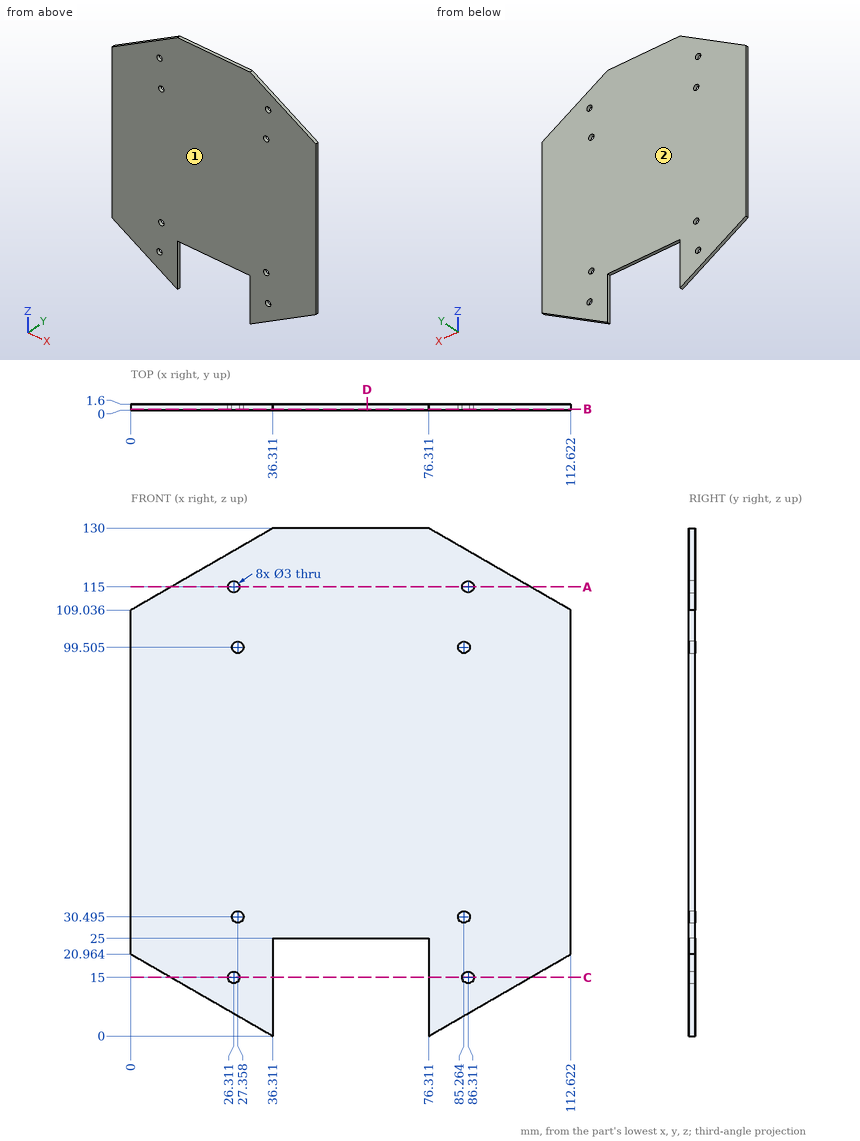
Check sheet for the drawn part. Datum: minimum x, y, z corner. Units: mm. Round coordinates to 2 decimals unless told otherwise and drop trailing zeros. Order: outer loops, then holes, each group sorted by start corner. A loop starts at its lowest first (then second) coordinate and runs counter-clockwise, first axis right, second up. Notation, with made-up numbers: (70.25, 5.5) - (82.25, 5.5) arc R22 cw to (82.25, 30.5) - close; hole circle Ø9 at (67.25, 0). An arc over 180 degrees is marked (long way). Use a Markdown table: item, result. Add a question column.
(1) Material ranges on line 1 along X through (y, z) = (1.25, 116); line 2 along X through (y, z) = (0.4, 115); line 3 along Z through (x, y) = (74.5, 0.9), recorded low to high. Write a range as [from, to].
(2) Sectioned sample at C-C, the plane z = 15. Enter the section's corners in (x, y).
(3) Release check for a two-part mould opening along Y. For the marked faces 1 and 2 record: pulls with the +Y half, pulls with the -Y half, needs draft (parallel to the pull), parting line crosses it, or undercut.
(4) Sectioned sample at D-D, the plane x = 60.5. Enter the section's corners in (y, z).
(5) Depth check by flat-ended pin: pin 1 (1.8 mm diameter, centred on x = 27.36, z = 99.5, fed in from +Y); pin 2 (0.8 mm diameter, centred on y = 1, z = 16, fed in from -X) (1 decimal); pin 3 (0.8 mm diameter, centred on y = 0.5, z = 16.5, fed in from +X). Enter the tip coordinate at first touch or a pass-through.
(6) Sectioned sample at A-A, the plane z = 115. Enter the section's corners in (x, y).
(7) Sectioned sample at B-B, the plane y = 0.3. Count the separate pieces of the cut face and the enclosed holes in it, and give its area (3 significant figures).
Answers below:
| question | item | result |
|---|---|---|
| 1 | line 1 | [12.06, 25.19], [27.43, 85.19], [87.43, 100.56] |
| 1 | line 2 | [10.33, 24.81], [27.81, 84.81], [87.81, 102.29] |
| 1 | line 3 | [25, 130] |
| 2 | outline | (10.33, 0) - (24.81, 0) - (24.81, 1.6) - (10.33, 1.6) - close; (27.81, 0) - (36.31, 0) - (36.31, 1.6) - (27.81, 1.6) - close; (76.31, 0) - (84.81, 0) - (84.81, 1.6) - (76.31, 1.6) - close; (87.81, 0) - (102.29, 0) - (102.29, 1.6) - (87.81, 1.6) - close |
| 3 | face 1 | pulls with the -Y half |
| 3 | face 2 | pulls with the +Y half |
| 4 | outline | (0, 25) - (1.6, 25) - (1.6, 130) - (0, 130) - close |
| 5 | pin 1 | through |
| 5 | pin 2 | x = 7.9 |
| 5 | pin 3 | x = 105.58 |
| 6 | outline | (10.33, 0) - (24.81, 0) - (24.81, 1.6) - (10.33, 1.6) - close; (27.81, 0) - (84.81, 0) - (84.81, 1.6) - (27.81, 1.6) - close; (87.81, 0) - (102.29, 0) - (102.29, 1.6) - (87.81, 1.6) - close |
| 7 | separate pieces | 1 |
| 7 | enclosed holes | 8 |
| 7 | area | 12,100 mm² |
